from build123d import *

# Parameters (mm, degrees)
ESQUISSE1_W             = 40
ESQUISSE1_H             = 17
BOSS_EXTRU_1_DEPTH      = 1
ENL_V_MAT_EXTRU_1_REACH = 45.474
ESQUISSE2_R             = 2.5
BOSS_EXTRU_2_DEPTH      = 8


with BuildPart() as part:
    # Esquisse1 → Boss.-Extru.1 (new body)
    with BuildSketch(Plane.XY):
        with Locations((20, 8.5)):
            Rectangle(ESQUISSE1_W, ESQUISSE1_H)
    extrude(amount=BOSS_EXTRU_1_DEPTH)

    # Esquisse2 → Enlèv. mat.-Extru.1 (cut, up to next)
    with BuildSketch(Plane.XY.offset(1), mode=Mode.PRIVATE) as enl_v_mat_extru_1_sk1:
        with Locations((6.5, 10.5)):
            Circle(ESQUISSE2_R)
    enl_v_mat_extru_1_tool1 = extrude(enl_v_mat_extru_1_sk1.sketch, amount=-ENL_V_MAT_EXTRU_1_REACH, mode=Mode.PRIVATE) & part.part
    # Esquisse2 → Enlèv. mat.-Extru.1 (cut, up to next)
    with BuildSketch(Plane.XY.offset(1), mode=Mode.PRIVATE) as enl_v_mat_extru_1_sk2:
        with Locations((33.5, 10.5)):
            Circle(ESQUISSE2_R)
    enl_v_mat_extru_1_tool2 = extrude(enl_v_mat_extru_1_sk2.sketch, amount=-ENL_V_MAT_EXTRU_1_REACH, mode=Mode.PRIVATE) & part.part
    add(enl_v_mat_extru_1_tool1.solids().sort_by_distance((6.5, 10.5, 1))[0], mode=Mode.SUBTRACT)
    add(enl_v_mat_extru_1_tool2.solids().sort_by_distance((33.5, 10.5, 1))[0], mode=Mode.SUBTRACT)

    # Esquisse3 → Boss.-Extru.2 (add)
    with BuildSketch(Plane.ZY.offset(-8)):
        with BuildLine():
            Line((0, 0), (0, -2))
            ThreePointArc((0, -2), (3.414213562, -3.414213562), (2, 0))
            Line((2, 0), (2, -1))
            ThreePointArc((2, -1), (2.707106781, -2.707106781), (1, -2))
            Line((1, -2), (1, 0))
            Line((1, 0), (0, 0))
        make_face()
    boss_extru_2 = extrude(amount=-BOSS_EXTRU_2_DEPTH)

    # Symétrie1: Boss.-Extru.2 across plane
    add(boss_extru_2.mirror(Plane.ZY.offset(-20)))


solid = part.part
The model under review builds one solid part; all positions refer to its coordinate system, in mm. A direction names the side the tool comes from. Give positions to 0.01 mm unless a question says otherwise; leave off trailing zeros. Loops run counter-clockwise (first coordinate to the right, second up) from the corner with the lowest first, then second, coordinate; pieces in that order, holes last. Notation, with made-up numbers: (33, 15) -> (85, 15) arc R33 ccw to (85, 47) -> close; hole circle Ø11 at (-19, 84.5). An arc over 180 degrees is marked (long way). Put each result on its own line as item: value. Start each with the question number.
1. Wall thickness on probe 1 along Y at (x, z) = (33.5, 0.7); probe 2 along Z at (x, y) = (26.5, -2); probe 3 along Z at (x, y) = (30, 5): over which ranges is each line inside the solid? List them lowest first.
2. Clearance check with flat-ended pins moving along their axes: P1, Ø2, axis at x = 30, y = 12.5, coming from the +Z side; P2, Ø0.8, axis at x = 3, z = 0.5, coming from the -Y side. State where each tip first meets the part, or that it passes through.
3. Mouldability with a two-part tool opening along X and no side actions: class faces 6 (the face through (40, 8.4, 0.5)), 7 (the face through (7.65, 8.28, 0.51)), 8 (the face through (28.056, -2.683, 2.73)) as released by +X, released by -X, zero draft, split by the parting line, or undercut.
4. We need section B-B on y = 10.5. State the section outline as (x, z) points, then the cut area to 3 significant figures.
5. We need section D-D on x = 24.5. State the section outline as (y, z) points, then the cut area to 3 significant figures.
6. We need section A-A on x = 33.5. State the section outline as (y, z) points.
7. For faces 1 (the face through (32, -3, 1)), 2 (the face through (8, -3, 1)), 3 (the face through (19.9, 0, 0.5)), 4 (the face through (28.1, -0.5, 2)), 5 (the face through (20, 8, 0)), list the 3-axis set-ups (+Z, -Z, +X, -X, +Y, -Y) from which the entire face can be reached by the end or side of a thin tool; tool diameter is ignored.
8. We need section C-C on z = 3.55. State the section outline as (x, y) points.
Determined:
1. probe 1: 0 to 8, 13 to 17
1. probe 2: 0 to 1, 3 to 4
1. probe 3: 0 to 1
2. P1: z = 1
2. P2: y = 0
3. face 6: released by +X
3. face 7: undercut
3. face 8: zero draft
4. outline: (0, 0) -> (4, 0) -> (4, 1) -> (0, 1) -> close; (9, 0) -> (31, 0) -> (31, 1) -> (9, 1) -> close; (36, 0) -> (40, 0) -> (40, 1) -> (36, 1) -> close
4. area: 30.0 mm^2
5. outline: (-2, 0) -> (17, 0) -> (17, 1) -> (-2, 1) arc R1 cw (long way) to (-1, 2) -> (0, 2) arc R2 ccw (long way) to start
5. area: 26.1 mm^2
6. outline: (0, 0) -> (8, 0) -> (8, 1) -> (0, 1) -> close; (13, 0) -> (17, 0) -> (17, 1) -> (13, 1) -> close
7. face 1: +Z, -Z, +X, -Y
7. face 2: +Z, -Z, -X, -Y
7. face 3: +Z, -Z, -Y
7. face 4: +X, -X, +Y
7. face 5: -Z, +X, -X, +Y, -Y
8. outline: (8, -3.26) -> (16, -3.26) -> (16, -0.74) -> (8, -0.74) -> close; (24, -3.26) -> (32, -3.26) -> (32, -0.74) -> (24, -0.74) -> close
